Geometry check sheet. Reference: the model listing, model coordinates, mm. Coordinates: 2 decimals unless noted, no trailing zeros. Write each loop counter-clockwise with the first axis right and the second up, starting at its lowest first coordinate (ties: lowest second). Pieces come first, ordered by that corner, then holes. Notation, with made-up numbers: (-19.75, 7) -> (20.25, 7) arc R9 ccw to (20.25, 12) -> close; hole circle Ø8 at (54, 19). An arc over 180 degrees is marked (long way). Use a Markdown table: item, result.
```python
from build123d import *

# Parameters (mm, degrees)
F1_DEPTH = 2400
F2_ANGLE = -110


with BuildPart() as f1:
    # F0 (on Front) → F1 (new body)
    with BuildSketch(Plane.XZ):
        with BuildLine():
            Line((28.5, 33.5), (-28.5, 33.5))
            ThreePointArc((-28.5, 33.5), (-32.035534, 32.035534), (-33.5, 28.5))
            Line((-33.5, 28.5), (-33.5, -28.5))
            ThreePointArc((-33.5, -28.5), (-32.035534, -32.035534), (-28.5, -33.5))
            Line((-28.5, -33.5), (28.5, -33.5))
            ThreePointArc((28.5, -33.5), (32.035534, -32.035534), (33.5, -28.5))
            Line((33.5, -28.5), (33.5, 28.5))
            ThreePointArc((33.5, 28.5), (32.035534, 32.035534), (28.5, 33.5))
        make_face()
    extrude(amount=F1_DEPTH)


with BuildPart() as f1_1:
    # F2: moved
    add(f1.part.rotate(Axis((0, 0, 33.5), (1, 0, 0)), F2_ANGLE))


with BuildPart() as f1_2:
    # F3: moved
    add(f1_1.part.moved(Location((0, -320, 0))))


solid = f1_2.part
```
Item 1: Section check A-A on x = -9. Record the boundary of the cut face in (y, z).
Answer block:
| item | result |
|---|---|
| outline | (-382.96, 56.42) -> (-320, 33.5) -> (500.85, 2288.76) -> (437.89, 2311.68) -> close |
Item 2: Depth check by flat-ended pin: P1, Ø8, axis at x = 12.5, z = 1030.5, coming from the -Y side; P2, Ø1, axis at x = -21, z = 1397, coming from the +Y side; P3, Ø2, axis at x = -16, z = 1606.5, coming from the -Y side. Enter the tip coordinate at first touch or a pass-through.
Answer block:
| item | result |
|---|---|
| P1 | stops at y = -29.88 |
| P2 | stops at y = 176.46 |
| P3 | stops at y = 180.86 |
Item 3: Thickness scan on L1, parallel to Y at x = 13, z = 1882; L2, parallel to Y at x = -3.5, z = 1024.5. Record the ranges inside material, lowest first. Write a range as [from, to].
Answer block:
| item | result |
|---|---|
| L1 | y = [281.5, 352.8] |
| L2 | y = [-30.61, 40.69] |
